Answer from the drawing. Dimensions are ordinates in mm from the lowest x, y and z of the part. A direction names the side the tool comes from. Give positions to 0.01 mm unless a question says otherwise; leave off trailing zeros. Write each loop counter-clockwise with the first axis right and the second up, starting at its lowest first coordinate (ties: lowest second). Pieces come first, ordered by that corner, then holes.
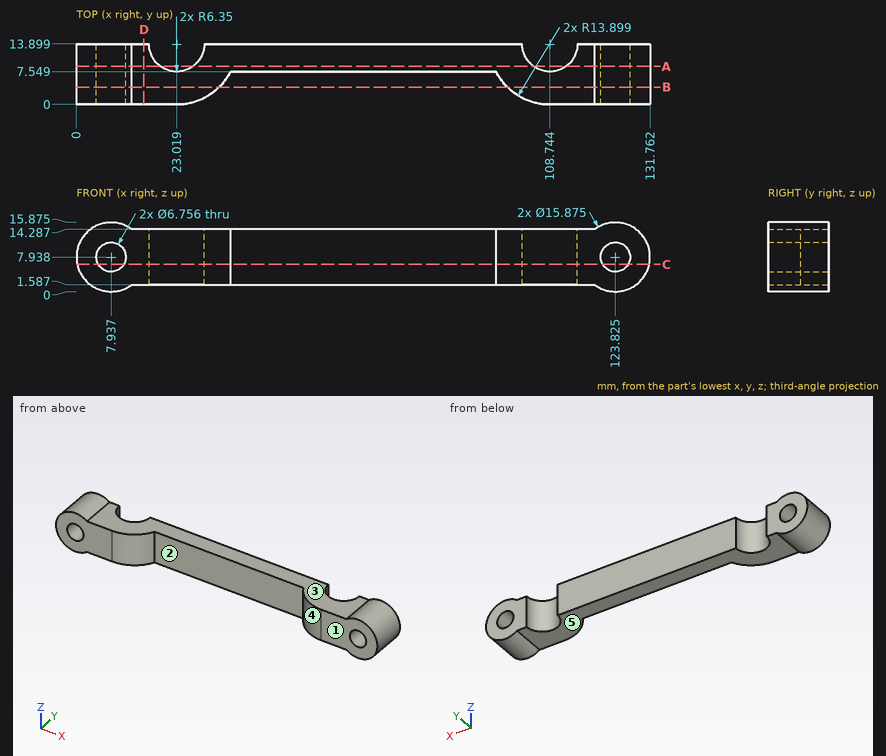
Item 1: Determine the mould class of the marked faces 1 and 2 for opening direction X: pulls with the +X half, pulls with the -X half, needs draft (parallel to the pull), parting line crosses it, or undercut.
Conclusion:
face 1: needs draft
face 2: undercut
Item 2: A cutting plane is placed at B-B, the plane y = 4. Give the vertices of the cut face in (x, z) (1 decimal).
Conclusion:
outline: (12.7, 1.6) - (32.8, 1.6) - (32.8, 14.3) - (12.7, 14.3) arc R7.9 ccw (long way) to start; (99, 1.6) - (119.1, 1.6) arc R7.9 ccw (long way) to (119.1, 14.3) - (99, 14.3) - close; hole circle Ø6.8 at (7.9, 7.9); hole circle Ø6.8 at (123.8, 7.9)
Item 3: A cutting plane is placed at C-C, the plane z = 6.25. Count the separate pieces of the cut face and the enclosed holes in it, plus the area to 3 significant figures.
Conclusion:
separate pieces: 3
enclosed holes: 0
area: 1,020 mm2
Item 4: Which of the six approach directions +Z, -Z, +X, -X, +Y, -Y give full straight-line access (tool end or side, diameter ignored) to the marked faces 3, 4 and 5?
Conclusion:
face 3: +Z, +Y, -Y
face 4: +Z, -Z, -Y
face 5: -Z, +Y, -Y
Item 5: Each of these flat-tipped pins is pushed along its axis until it touches: P1, Ø2, axis at x = 30.5, y = 6.5, coming from the -Z side; P2, Ø2, axis at x = 74, y = 10, coming from the +Z side; P3, Ø4, axis at x = 7.94, z = 7.94, coming from the +Y side (3 decimals); P4, Ø1.5, axis at x = 55.5, z = 7, coming from the -Y side. Where does it stop, or does it pass through?
Conclusion:
P1: stops at z = 1.59
P2: stops at z = 14.29
P3: passes through
P4: stops at y = 7.55
Item 6: A cutting plane is placed at D-D, the plane x = 15.5. Give the vertices of the cut face in (y, z).
Conclusion:
outline: (0, 1.59) - (13.9, 1.59) - (13.9, 14.29) - (0, 14.29) - close
Item 7: Consider probe 1 along X at (y, z) = (5.75, 0.75) (1 decimal); probe 2 along Z at (x, y) = (115, 4.5); probe 3 along Y at (x, z) = (109, 12.75) (1 decimal). Determine where each line is inside the solid, lowest interval first.
Conclusion:
probe 1: x = 4.6 to 11.3, 120.5 to 127.2
probe 2: z = 1.59 to 14.29
probe 3: y = 0 to 7.6
Item 8: A cutting plane is placed at A-A, the plane y = 8.75. Give the vertices of the cut face in (x, z) (1 decimal), plus the area to 3 significant figures.
Conclusion:
outline: (12.7, 1.6) - (19.3, 1.6) - (19.3, 14.3) - (12.7, 14.3) arc R7.9 ccw (long way) to start; (26.7, 1.6) - (105, 1.6) - (105, 14.3) - (26.7, 14.3) - close; (112.5, 1.6) - (119.1, 1.6) arc R7.9 ccw (long way) to (119.1, 14.3) - (112.5, 14.3) - close; hole circle Ø6.8 at (7.9, 7.9); hole circle Ø6.8 at (123.8, 7.9)
area: 1,430 mm2
